Solid Edge part; units mm, degrees
sketch "Sketch1" plane through (0, 0, 0) normal (0, -1, 0) x (1, 0, 0)
  line L0 (-2.4, 95) -> (2.4, 95)
  line L1 (2.4, 95) -> (2.4, 30)
  line L2 (2.4, 30) -> (-2.4, 30)
  line L3 (-2.4, 30) -> (-2.4, 95)
  dimension "D1" = 2.4
revolve "RevolvedProtrusion1" add sketch "Sketch1" angle 360 about axis through (-60, 0, 0) along (1, 0, 0)
hole "Hole1" at (2.4, 0, 45) direction (-1, 0, 0) diameter 9 end up to next
pattern_circular "Pattern1" count 6 over 360 about axis through (2.4, 0, 0) along (-1, 0, 0) of "Hole1"
properties material "Stainless Steel, 420"
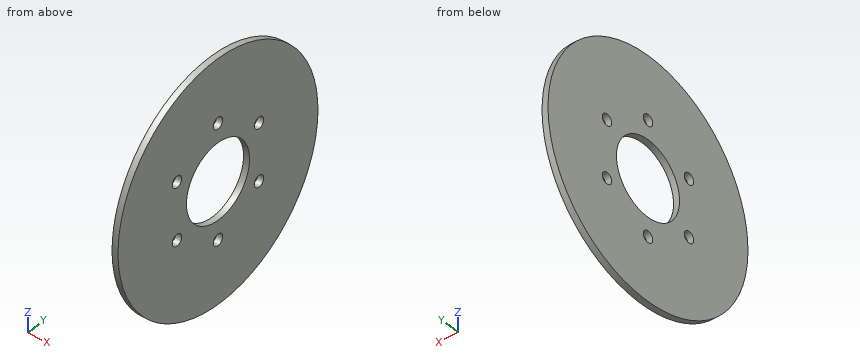
Here's how the part is built. I have some questions about the finished solid (model axes, mm). Coordinates: 2 decimals unless noted, no trailing zeros. Order: outer loops, then holes, each group sorted by start corner. A loop starts at its lowest first (then second) coordinate and runs counter-clockwise, first axis right, second up. Notation, with made-up numbers: M 23.25,69 L 49.25,69 A11 ccw 49.25,81 Z; hole C 42,59 d10. An arc over 180 degrees is marked long. Answer as CSV lines item,"result". Start each with the question number.
1. I want a section at A-A, the plane y = 0. Write out the boundary of the cut face in (x, z), and give its area (3 significant figures).
2. I want a section at B-B, the plane z = 0. Write out the boundary of the cut face in (x, y).
3. I need wall thicknesses on line 1 (Z direction, x = 0.6, y = 0); line 2 (Y direction, x = -1.2, z = 0); line 3 (Z direction, x = 0.4, y = -3.5). Which ranges of each line are inside material? Lowest first, please. Write a range as [from, to].
4. I want a section at C-C, the plane x = -0.75. Write out the boundary of the cut face in (y, z).
5. For pin 1 (7 mm diameter, centred on y = -38.97, z = -22.5, fed in from -X); pin 2 (1 mm diameter, centred on x = 0, y = -49, fed in from +Z); pin 3 (1.5 mm diameter, centred on x = 1, z = -27, fed in from -Y), each with a flat end and sliding along its axis, tell me the tip position at first contact or that it passes through.
6. I want a section at D-D, the plane z = -22.5. Write out the boundary of the cut face in (x, y).
Recorded:
1,outline,"M -2.4,-95 L 2.4,-95 L 2.4,-49.5 L -2.4,-49.5 Z; M -2.4,-40.5 L 2.4,-40.5 L 2.4,-30 L -2.4,-30 Z; M -2.4,30 L 2.4,30 L 2.4,40.5 L -2.4,40.5 Z; M -2.4,49.5 L 2.4,49.5 L 2.4,95 L -2.4,95 Z"
1,area,"538 mm2"
2,outline,"M -2.4,-95 L 2.4,-95 L 2.4,-30 L -2.4,-30 Z; M -2.4,30 L 2.4,30 L 2.4,95 L -2.4,95 Z"
3,line 1,"z = [-95, -49.5], [-40.5, -30], [30, 40.5], [49.5, 95]"
3,line 2,"y = [-95, -30], [30, 95]"
3,line 3,"z = [-94.94, -47.83], [-42.17, -29.8], [29.8, 42.17], [47.83, 94.94]"
4,outline,"C 0,0 d190; hole C -38.97,-22.5 d9; hole C -38.97,22.5 d9; hole C 0,0 d60; hole C 0,-45 d9; hole C 0,45 d9; hole C 38.97,-22.5 d9; hole C 38.97,22.5 d9"
5,pin 1,"passes through"
5,pin 2,"stops at z = 81.69"
5,pin 3,"stops at y = -91.3"
6,outline,"M -2.4,-92.3 L 2.4,-92.3 L 2.4,-43.47 L -2.4,-43.47 Z; M -2.4,-34.47 L 2.4,-34.47 L 2.4,-19.84 L -2.4,-19.84 Z; M -2.4,19.84 L 2.4,19.84 L 2.4,34.47 L -2.4,34.47 Z; M -2.4,43.47 L 2.4,43.47 L 2.4,92.3 L -2.4,92.3 Z"
